from build123d import *

# Parameters (mm, degrees)
SKETCH1_R           = 3.3782
BOSS_EXTRUDE1_DEPTH = 9.525
SKETCH3_W           = 9.652
SKETCH3_H           = 25.4
CUT_EXTRUDE1_DEPTH  = 68.594698618


with BuildPart() as part:
    # Sketch1 → Boss-Extrude1 (new, symmetric)
    with BuildSketch(Plane.XY):
        Polygon((-12.7, 23.8125), (-12.7, 36.5125), (12.7, 36.5125), (12.7, 23.8125), (12.7, -61.9125), (-12.7, -61.9125), align=None)
        with Locations(Location((0, 23.8125, 0), (0, 0, 180))):
            Circle(SKETCH1_R, mode=Mode.SUBTRACT)
        with Locations(Location((0, -23.8125, 0), (0, 0, 180))):
            Circle(SKETCH1_R, mode=Mode.SUBTRACT)
    extrude(amount=BOSS_EXTRUDE1_DEPTH, both=True)

    # Sketch3 → Cut-Extrude1 (cut, through all)
    with BuildSketch(Plane(origin=(12.7, 0, 0), x_dir=(0, 0, -1), z_dir=(1, 0, 0))):
        with Locations((0, 23.8125)):
            Rectangle(SKETCH3_W, SKETCH3_H)
    extrude(amount=-CUT_EXTRUDE1_DEPTH, mode=Mode.SUBTRACT)


solid = part.part
Read the model definition and answer for the solid it produces. Units are mm, in the model's axes. A direction names the side the tool comes from. Give positions to 0.01 mm unless a question says otherwise; leave off trailing zeros. Loops run counter-clockwise (first coordinate to the right, second up) from the corner with the lowest first, then second, coordinate; pieces in that order, holes last. Notation, with made-up numbers: (-27.5, 53) - (-16.5, 53) arc R18 ccw to (-16.5, 86) - close; hole circle Ø2 at (-15.75, 36.5). An arc over 180 degrees is marked (long way). Answer as CSV lines item,"result". Start each with the question number.
1) Each of these flat-tipped pins is pushed along its axis until it touches: pin 1 Ø5.5 at (x, y) = (0, 23.81) entering from -Z; pin 2 Ø3 at (x, z) = (-5.5, 0.5) entering from +Y. Where does it stop, or does it pass through?
2) Find section D-D (z = 3.25). Write down the section's boundary in (x, y).
3) Straight lines are drawn through the part: L1, parallel to Y at x = 0, z = -6.6; L2, parallel to Y at x = 0, z = -3.75; L3, parallel to Z at x = -10.25, y = 20.5 (3 decimals). For each, find the intervals that lie inside material, in ascending order. Write a range as from..to.
4) Determine the mould class of faces 1 (the face through (0, -12, 9.525)), 2 (the face through (0, -61.912, 0)), 3 (the face through (3, 26, 4.826)), 4 (the face through (0, -12, -9.525)) for opening direction Z: released by +Z, released by -Z, zero draft, split by the parting line, or undercut.
5) Find section C-C (x = -7). Write down the section's boundary in (y, z) (1 decimal).
6) Which of the six approach directions +Z, -Z, +X, -X, +Y, -Y give full straight-line access (tool end or side, diameter ignored) to faces 5 (the face through (-12.7, -12, 0)), 6 (the face through (0, 11.112, 0))?
7) Find section B-B (x = 0). Write down the section's boundary in (y, z) (1 decimal).
8) Find section A-A (y = 30.5). Write down the section's boundary in (x, z) (3 decimals).
Findings below:
1,pin 1,"through"
1,pin 2,"y = 11.11"
2,outline,"(-12.7, -61.91) - (12.7, -61.91) - (12.7, 11.11) - (-12.7, 11.11) - close; hole circle Ø6.76 at (0, -23.81)"
3,L1,"-61.91..-27.19, -20.43..20.43, 27.19..36.51"
3,L2,"-61.91..-27.19, -20.43..11.11"
3,L3,"-9.525..-4.826, 4.826..9.525"
4,face 1,"released by +Z"
4,face 2,"zero draft"
4,face 3,"undercut"
4,face 4,"released by -Z"
5,outline,"(-61.9, -9.5) - (36.5, -9.5) - (36.5, -4.8) - (11.1, -4.8) - (11.1, 4.8) - (36.5, 4.8) - (36.5, 9.5) - (-61.9, 9.5) - close"
6,face 5,"+Z, -Z, -X, +Y, -Y"
6,face 6,"+X, -X, +Y"
7,outline,"(-61.9, -9.5) - (-27.2, -9.5) - (-27.2, 9.5) - (-61.9, 9.5) - close; (-20.4, -9.5) - (20.4, -9.5) - (20.4, -4.8) - (11.1, -4.8) - (11.1, 4.8) - (20.4, 4.8) - (20.4, 9.5) - (-20.4, 9.5) - close; (27.2, -9.5) - (36.5, -9.5) - (36.5, -4.8) - (27.2, -4.8) - close; (27.2, 4.8) - (36.5, 4.8) - (36.5, 9.5) - (27.2, 9.5) - close"
8,outline,"(-12.7, -9.525) - (12.7, -9.525) - (12.7, -4.826) - (-12.7, -4.826) - close; (-12.7, 4.826) - (12.7, 4.826) - (12.7, 9.525) - (-12.7, 9.525) - close"
